For this review, use the dimensioned drawing (mm, ordinates from the lowest corner) and the shaded views. A direction names the side the tool comes from. Round coordinates to 2 decimals unless told otherwise and drop trailing zeros. Order: outer loops, then holes, each group sorted by start corner. A loop starts at its lowest first (then second) coordinate and runs counter-clockwise, first axis right, second up. Notation, with made-up numbers: (17.5, 52) - (38.5, 52) arc R22 cw to (38.5, 91) - close; hole circle Ø2 at (55.5, 64.25). An arc over 180 degrees is marked (long way). Write item = value, one per line.
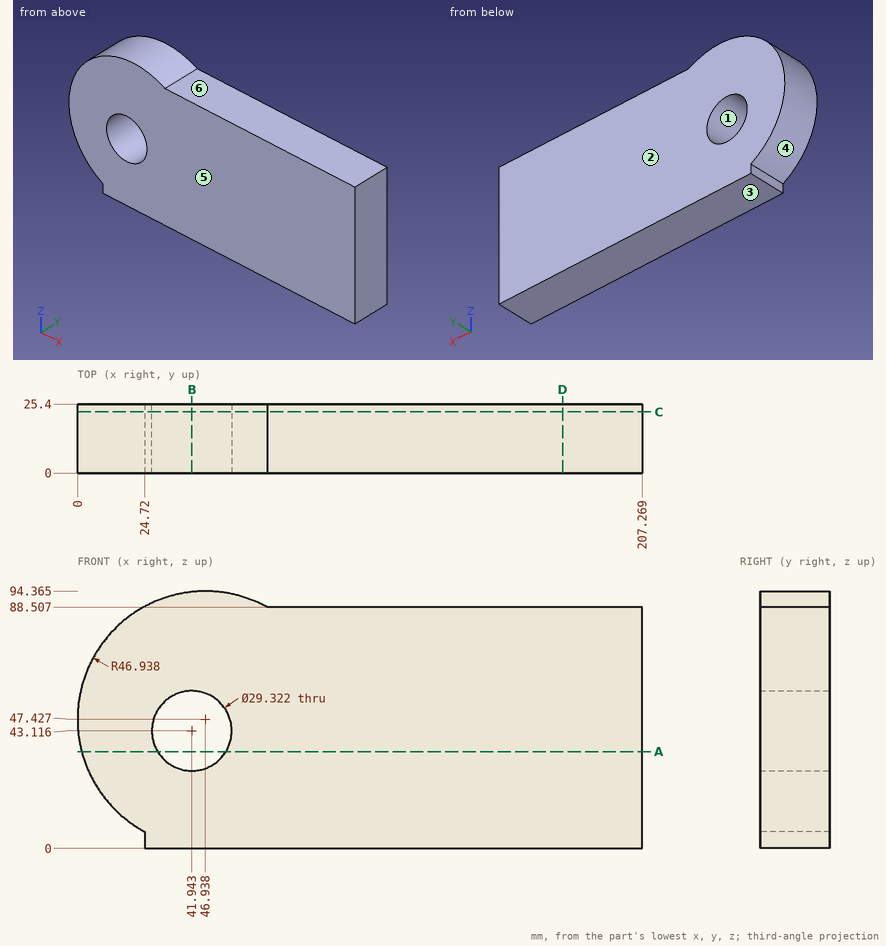
1) We need section D-D on x = 178. Write out the cut boundary in (y, z).
Findings:
outline = (0, 0) - (25.4, 0) - (25.4, 88.51) - (0, 88.51) - close
2) The part is to be moulded in two halves that separate along Z. For the marked faces 1, 2, 3 and 4, say which applies: released by +Z, released by -Z, zero draft, split by the parting line, or undercut.
Findings:
face_1 = undercut
face_2 = zero draft
face_3 = released by -Z
face_4 = split by the parting line
3) For the marked faces 5 and 6, list the 3-axis set-ups (+Z, -Z, +X, -X, +Y, -Y) from which the entire face can be reached by the end or side of a thin tool; tool diameter is ignored.
Findings:
face_5 = +Z, -Z, +X, -X, -Y
face_6 = +Z, +X, +Y, -Y
4) We need section B-B on x = 42. Write out the cut boundary in (y, z) (1 decimal), and give its area (3 significant figures).
Findings:
outline = (0, 0) - (25.4, 0) - (25.4, 28.5) - (0, 28.5) - close; (0, 57.8) - (25.4, 57.8) - (25.4, 94.1) - (0, 94.1) - close
area = 1,650 mm^2
5) Clearance check with flat-ended pins moving along their axes: pin 1 Ø1.5 at (x, y) = (132, 19.5) entering from +Z; pin 2 Ø6 at (y, z) = (13.5, 68.5) entering from -X; pin 3 Ø3 at (y, z) = (7, 4) entering from -X. State where each tip first meets the part, or that it passes through.
Findings:
pin_1 = 88.51
pin_2 = 3.62
pin_3 = 24.72
6) We need section C-C on y = 22.5. Write out the cut boundary in (x, z) (1 decimal), and give its area (3 significant figures).
Findings:
outline = (24.7, 0) - (207.3, 0) - (207.3, 88.5) - (69.6, 88.5) arc R46.9 ccw (long way) to (24.7, 6.1) - close; hole circle Ø29.3 at (41.9, 43.1)
area = 17,100 mm^2
7) To check wall thickness, follow L1, parallel to Z at x = 158, y = 12.5; L2, parallel to X at y = 23.5, z = 37.5 (1 decimal); L3, parallel to X at y = 11.5, z = 30 (1 decimal). State the ranges of each line that lie inside material, in increasing order. Write a range as from..to.
Findings:
L1 = 0..88.51
L2 = 1.1..28.4, 55.5..207.3
L3 = 3.4..35.4, 48.5..207.3
8) We need section A-A on z = 35.5. Write out the cut boundary in (x, y) (1 decimal).
Findings:
outline = (1.5, 0) - (29.4, 0) - (29.4, 25.4) - (1.5, 25.4) - close; (54.5, 0) - (207.3, 0) - (207.3, 25.4) - (54.5, 25.4) - close
